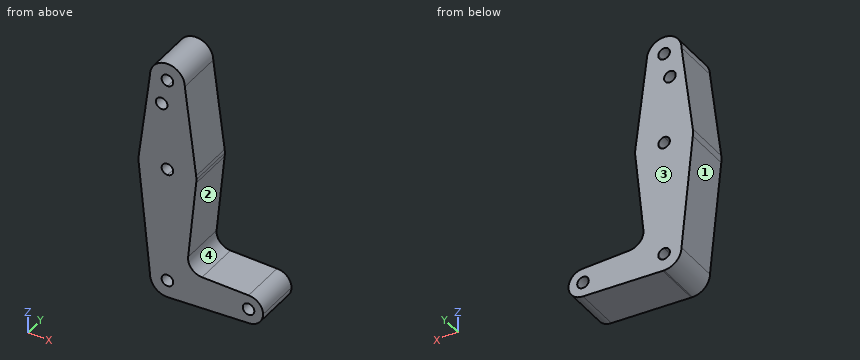
from build123d import *

# Parameters (mm, degrees)
F0_R     = 3.175
F1_DEPTH = 25.4


with BuildPart() as f1:
    # F0 (on Front) → F1 (new body)
    with BuildSketch(Plane.XZ):
        with BuildLine():
            ThreePointArc((0, 9.525), (-6.7351920908, 6.7351920908), (-9.525, 0))
            ThreePointArc((-9.525, 0), (-6.7351920908, -6.7351920908), (0, -9.525))
            Line((0, -9.525), (0.6794904459, -9.5007324841))
            ThreePointArc((0.6794904459, -9.5007324841), (6.9712901065, -6.4905114784), (9.525, 0))
            Line((9.525, 0), (3.175, 0))
            ThreePointArc((3.175, 0), (-2.2450640303, -2.2450640303), (0, 3.175))
            Line((0, 3.175), (0, 9.525))
        make_face()
        with BuildLine():
            Line((-15.7474569047, 61.4917106696), (-9.525, 0))
            ThreePointArc((-9.525, 0), (-6.7351920908, 6.7351920908), (0, 9.525))
            Line((0, 9.525), (0, 47.625))
            ThreePointArc((0, 47.625), (-10.4912828548, 51.5857812233), (-15.7474569047, 61.4917106696))
        make_face()
        with BuildLine():
            Line((0.6794904459, -9.5007324841), (0, -9.525))
            ThreePointArc((0, -9.525), (0.3399618281, -9.5189311877), (0.6794904459, -9.5007324841))
        make_face()
        with BuildLine():
            Line((0, 47.625), (0, 9.525))
            ThreePointArc((0, 9.525), (6.7351920908, 6.7351920908), (9.525, 0))
            Line((9.525, 0), (36.5125, 0))
            ThreePointArc((36.5125, 0), (38.8373399243, 5.6126600757), (44.45, 7.9375))
            Line((44.45, 7.9375), (18.9647942191, 8.8511945514))
            ThreePointArc((18.9647942191, 8.8511945514), (13.2592410586, 11.5693613748), (11.3392208, 17.5905979549))
            Line((11.3392208, 17.5905979549), (15.7474569047, 61.4917106696))
            ThreePointArc((15.7474569047, 61.4917106696), (10.4912828548, 51.5857812233), (0, 47.625))
        make_face()
        with BuildLine():
            ThreePointArc((-15.7474569047, 65.5082893304), (-15.875, 63.5), (-15.7474569047, 61.4917106696))
            ThreePointArc((-15.7474569047, 61.4917106696), (-10.4912828548, 51.5857812233), (0, 47.625))
            Line((0, 47.625), (0, 60.325))
            ThreePointArc((0, 60.325), (-3.175, 63.5), (0, 66.675))
            Line((0, 66.675), (0, 79.375))
            ThreePointArc((0, 79.375), (-10.4912828548, 75.4142187767), (-15.7474569047, 65.5082893304))
        make_face()
        with BuildLine():
            ThreePointArc((9.525, 0), (6.9712901065, -6.4905114784), (0.6794904459, -9.5007324841))
            Line((0.6794904459, -9.5007324841), (44.45, -7.9375))
            ThreePointArc((44.45, -7.9375), (38.8373399243, -5.6126600757), (36.5125, 0))
            Line((36.5125, 0), (9.525, 0))
        make_face()
        with BuildLine():
            Line((0, 60.325), (0, 47.625))
            ThreePointArc((0, 47.625), (10.4912828548, 51.5857812233), (15.7474569047, 61.4917106696))
            ThreePointArc((15.7474569047, 61.4917106696), (15.8430821396, 62.4938323604), (15.875, 63.5))
            ThreePointArc((15.875, 63.5), (15.8430821396, 64.5061676396), (15.7474569047, 65.5082893304))
            ThreePointArc((15.7474569047, 65.5082893304), (10.4912828548, 75.4142187767), (0, 79.375))
            Line((0, 79.375), (0, 66.675))
            ThreePointArc((0, 66.675), (2.2450640303, 65.7450640303), (3.175, 63.5))
            ThreePointArc((3.175, 63.5), (2.2450640303, 61.2549359697), (0, 60.325))
        make_face()
        with BuildLine():
            Line((-9.525, 114.3), (-15.7474569047, 65.5082893304))
            ThreePointArc((-15.7474569047, 65.5082893304), (-10.4912828548, 75.4142187767), (0, 79.375))
            Line((0, 79.375), (0, 100.0252))
            Line((0, 100.0252), (0, 104.775))
            ThreePointArc((0, 104.775), (-6.7351920908, 107.5648079092), (-9.525, 114.3))
        make_face()
        with Locations((-3.175, 100.0252)):
            Circle(F0_R, mode=Mode.SUBTRACT)
        with BuildLine():
            ThreePointArc((36.5125, 0), (38.8373399243, -5.6126600757), (44.45, -7.9375))
            ThreePointArc((44.45, -7.9375), (50.0626600757, -5.6126600757), (52.3875, 0))
            ThreePointArc((52.3875, 0), (50.0626600757, 5.6126600757), (44.45, 7.9375))
            ThreePointArc((44.45, 7.9375), (38.8373399243, 5.6126600757), (36.5125, 0))
        make_face()
        with BuildLine():
            ThreePointArc((47.625, 0), (44.45, -3.175), (41.275, 0))
            ThreePointArc((41.275, 0), (44.45, 3.175), (47.625, 0))
        make_face(mode=Mode.SUBTRACT)
        with BuildLine():
            Line((0, 100.0252), (0, 79.375))
            ThreePointArc((0, 79.375), (10.4912828548, 75.4142187767), (15.7474569047, 65.5082893304))
            Line((15.7474569047, 65.5082893304), (9.525, 114.3))
            ThreePointArc((9.525, 114.3), (6.7351920908, 107.5648079092), (0, 104.775))
            Line((0, 104.775), (0, 100.0252))
        make_face()
        with BuildLine():
            ThreePointArc((9.525, 114.3), (0, 123.825), (-9.525, 114.3))
            ThreePointArc((-9.525, 114.3), (-6.7351920908, 107.5648079092), (0, 104.775))
            ThreePointArc((0, 104.775), (6.7351920908, 107.5648079092), (9.525, 114.3))
        make_face()
        with BuildLine():
            ThreePointArc((3.175, 114.3), (2.2450640303, 112.0549359697), (0, 111.125))
            ThreePointArc((0, 111.125), (-2.2450640303, 116.5450640303), (3.175, 114.3))
        make_face(mode=Mode.SUBTRACT)
        with BuildLine():
            ThreePointArc((9.525, 0), (6.7351920908, 6.7351920908), (0, 9.525))
            Line((0, 9.525), (0, 3.175))
            ThreePointArc((0, 3.175), (2.2450640303, 2.2450640303), (3.175, 0))
            Line((3.175, 0), (9.525, 0))
        make_face()
    extrude(amount=F1_DEPTH)


solid = f1.part
Model file for the job. Use its own axes, mm. Face numbers are marked on the shaded views. Round coordinates to 2 decimals unless told otherwise and drop trailing zeros. Loops run counter-clockwise (first coordinate to the right, second up) from the corner with the lowest first, then second, coordinate; pieces in that order, holes last. Notation, with made-up numbers: (25.25, -5.5) -> (67.25, -5.5) arc R33 cw to (67.25, 30.5) -> close; hole circle Ø6 at (34, 61). An arc over 180 degrees is marked (long way). Answer as CSV lines item,"result". Start each with the question number.
1) Pin check, flat tips, straight feed: P1, Ø6, axis at x = 3.5, y = -7.5, coming from the -Z side; P2, Ø8, axis at x = 5, y = -15, coming from the +Z side; P3, Ø1, axis at y = -18, z = 8, coming from the -X side. Stop position of each tip, or through.
2) Slice it at C-C (x = 30). List the corners of the cut face in (y, z), plus the area to 3 significant figures.
3) Slice it at A-A (y = -5). State how many separate pieces and enclosed holes the cut face has, plus the area to 3 significant figures.
4) Mould opens along Z. For the marked faces 1, 2, 3 and 4 say: +Z half, -Z half, draft (parallel to the pull), parting line (faces both ways), or undercut.
5) Probe line 1 along Z through (x, y) = (-1, -15.25); line 2 along Z through (x, y) = (-1.5, -6.5); line 3 along X through (y, z) = (-15.5, 114.3) (3 decimals). List the from-to ranges inside material, lowest first.
6) Slice it at B-B (z = 70.5). List the corners of the cut face in (x, y).
Filled in:
1,P1,"stops at z = -9.51"
1,P2,"stops at z = 123.77"
1,P3,"stops at x = -10.39"
2,outline,"(-25.4, -8.45) -> (0, -8.45) -> (0, 8.46) -> (-25.4, 8.46) -> close"
2,area,"429 mm2"
3,separate pieces,"1"
3,enclosed holes,"5"
3,area,"3,770 mm2"
4,face 1,"-Z half"
4,face 2,"undercut"
4,face 3,"draft"
4,face 4,"undercut"
5,line 1,"z = -9.47 to -3.01, 3.01 to 60.49, 66.51 to 97.71, 102.34 to 111.29, 117.31 to 123.77"
5,line 2,"z = -9.41 to -2.8, 2.8 to 60.7, 66.3 to 97.33, 102.72 to 111.5, 117.1 to 123.71"
5,line 3,"x = -9.525 to -3.175, 3.175 to 9.525"
6,outline,"(-15.11, -25.4) -> (15.11, -25.4) -> (15.11, 0) -> (-15.11, 0) -> close"
